```python
from build123d import *

# Parameters (mm, degrees)
PAD002_DEPTH = 9.8
SKETCH008_R  = 1
PAD003_DEPTH = 4
SKETCH009_R  = 1
PAD004_DEPTH = 4


with BuildPart() as part:
    # Sketch006 → Pad002 (new body, symmetric)
    with BuildSketch(Plane.YZ):
        with BuildLine():
            Line((12.2, 2), (-12.2, 2))
            Line((-12.2, 2), (-12.2, 4.047819))
            ThreePointArc((12.2, 4.12971), (-0.003057, 4.999537), (-12.2, 4.047819))
            Line((12.2, 2), (12.2, 4.12971))
        make_face()
    extrude(amount=PAD002_DEPTH, both=True)

    # Sketch008 → Pad003 (new body)
    with BuildSketch(Plane.YZ.offset(9.8)):
        with Locations((6.5, 3.3)):
            Circle(SKETCH008_R)
    extrude(amount=PAD003_DEPTH)

    # Sketch009 → Pad004 (new body)
    with BuildSketch(Plane(origin=(-9.8, 0, 0), x_dir=(0, 1, 0), z_dir=(-1, 0, 0))):
        with Locations((6.5, -3.3)):
            Circle(SKETCH009_R)
    extrude(amount=PAD004_DEPTH)


solid = part.part
```
The model under review builds one solid part; all positions refer to its coordinate system, in mm. A direction names the side the tool comes from. Round coordinates to 2 decimals unless told otherwise and drop trailing zeros. Order: outer loops, then holes, each group sorted by start corner. A loop starts at its lowest first (then second) coordinate and runs counter-clockwise, first axis right, second up.
Item 1: Add section B-B, the plane y = 6.5. State the section outline as (x, z) points.
Working result:
outline: (-13.8, 2.3) - (-9.8, 2.3) - (-9.8, 2) - (9.8, 2) - (9.8, 2.3) - (13.8, 2.3) - (13.8, 4.3) - (9.8, 4.3) - (9.8, 4.76) - (-9.8, 4.76) - (-9.8, 4.3) - (-13.8, 4.3) - close
Item 2: Machinability: for faces 1 (the cylindrical face through (-11.772, 5.763, 2.624)), 2 (the cylindrical face through (11.8, 5.7, 2.7)), 3 (the flat face through (0, -12.2, 3)), which of the approach directions +Z, -Z, +X, -X, +Y, -Y give a long, thin tool a straight path to every point of the face, cutting with its end or side? Answer none if there is none.
Working result:
face 1: -X
face 2: +X
face 3: +Z, -Z, +X, -X, -Y
Item 3: Add section C-C, the plane x = 3. State the section outline as (y, z) points, and give its area (3 significant figures).
Working result:
outline: (-12.2, 2) - (12.2, 2) - (12.2, 4.13) arc R82.17 ccw to (-12.2, 4.05) - close
area: 65.8 mm2
Item 4: Add section D-D, the plane y = -10.25. State the section outline as (x, z) points, and give its area (3 significant figures).
Working result:
outline: (-9.8, 2) - (9.8, 2) - (9.8, 4.32) - (-9.8, 4.32) - close
area: 45.5 mm2
Item 5: To check wall thickness, follow probe 1 along X at (y, z) = (-4.5, 2.65); probe 2 along Y at (x, z) = (-11.5, 3.2); probe 3 along Z at (x, y) = (-12, 5.75). State the ranges of each line that lie inside material, in increasing order.
Working result:
probe 1: x = -9.8 to 9.8
probe 2: y = 5.51 to 7.49
probe 3: z = 2.64 to 3.96
Item 6: Add section A-A, the plane z = 3.3. State the section outline as (x, y) points, and give its area (3 significant figures).
Working result:
outline: (-13.8, 5.5) - (-9.8, 5.5) - (-9.8, -12.2) - (9.8, -12.2) - (9.8, 5.5) - (13.8, 5.5) - (13.8, 7.5) - (9.8, 7.5) - (9.8, 12.2) - (-9.8, 12.2) - (-9.8, 7.5) - (-13.8, 7.5) - close
area: 494 mm2
Item 7: For pin 1 (1 mm diameter, centred on y = -1, z = 3.5, fed in from -X); pin 2 (4 mm diameter, centred on x = 9, y = 8, fed in from +Z); pin 3 (0.9 mm diameter, centred on y = 0.5, z = 3, fed in from +X), all flat-tipped, find the tip position at first contact; note any pin that passes through.
Working result:
pin 1: stops at x = -9.8
pin 2: stops at z = 4.8
pin 3: stops at x = 9.8
